Could you check a few things on this drawing? It's one solid part, dimensions in mm from its lowest x, y, z. A direction names the side the tool comes from. Round coordinates to 2 decimals unless told otherwise and drop trailing zeros. Write each loop counter-clockwise with the first axis right and the second up, starting at its lowest first coordinate (ties: lowest second). Pieces come first, ordered by that corner, then holes. Notation, with made-up numbers: (-21.75, 16) -> (24.25, 16) arc R27 cw to (24.25, 38) -> close; hole circle Ø4 at (63.25, 49). An arc over 180 degrees is marked (long way). Answer in a Markdown table with one row per item.
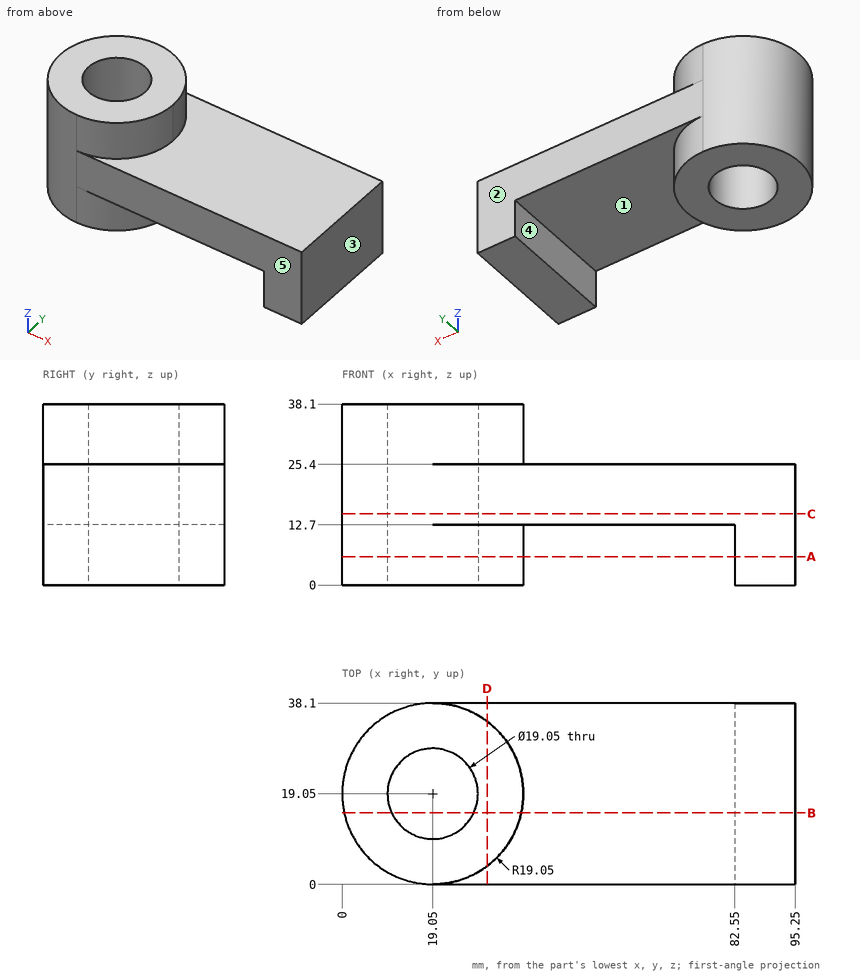
1) Please list where these lines run through material, in increasing order: line 1 (X direction, y = 19, z = 11); line 2 (Y direction, x = 19, z = 25); line 3 (X direction, y = 15, z = 3.5).
Findings:
| item | result |
|---|---|
| line 1 | x = 0 to 9.53, 28.57 to 38.1, 82.55 to 95.25 |
| line 2 | y = 0 to 9.53, 28.57 to 38.1 |
| line 3 | x = 0.44 to 10.43, 27.67 to 37.66, 82.55 to 95.25 |
2) Imagine slicing it at D-D, the plane x = 30.5. Please give me the cut outline in (y, z).
Findings:
| item | result |
|---|---|
| outline | (0, 12.7) -> (3.83, 12.7) -> (3.83, 0) -> (34.27, 0) -> (34.27, 12.7) -> (38.1, 12.7) -> (38.1, 25.4) -> (34.27, 25.4) -> (34.27, 38.1) -> (3.83, 38.1) -> (3.83, 25.4) -> (0, 25.4) -> close |
3) Imagine slicing it at C-C, the plane z = 15. Please give me the cut outline in (x, y) (3 decimals), plus the area to 3 significant figures.
Findings:
| item | result |
|---|---|
| outline | (19.05, 0) -> (95.25, 0) -> (95.25, 38.1) -> (19.05, 38.1) arc R19.05 ccw to start; hole circle Ø19.05 at (19.05, 19.05) |
| area | 3,190 mm^2 |
4) For pin 1 (4 mm diameter, centred on y = 28, z = 7, fed in from -X); pin 2 (5 mm diameter, centred on y = 5, z = 24, fed in from -X); pin 3 (3 mm diameter, centred on y = 26.5, z = 25.5, fed in from -X), each with a flat end and sliding along its axis, tell me the tip position at first contact or that it passes through.
Findings:
| item | result |
|---|---|
| pin 1 | stops at x = 1.31 |
| pin 2 | stops at x = 3.9 |
| pin 3 | stops at x = 0.95 |
5) Imagine slicing it at A-A, the plane z = 6. Please give me the cut outline in (x, y) (3 decimals).
Findings:
| item | result |
|---|---|
| outline | (19.05, 0) arc R19.05 ccw to (38.1, 19.05) arc R19.05 ccw (long way) to start; (82.55, 0) -> (95.25, 0) -> (95.25, 38.1) -> (82.55, 38.1) -> close; hole circle Ø19.05 at (19.05, 19.05) |
6) For the marked faces 4 and 5, which set-ups out of +Z, -Z, +X, -X, +Y, -Y let a thin tool reach every point of the face, with its end or its side?
Findings:
| item | result |
|---|---|
| face 4 | -Z, +Y, -Y |
| face 5 | +Z, -Z, +X, -X, -Y |
7) Thinking about a two-plate mould opening in X: for the marked faces 1, 2 and 3, which applies, +X half, -X half, draft (parallel to the pull), parting line (faces both ways), or undercut?
Findings:
| item | result |
|---|---|
| face 1 | undercut |
| face 2 | draft |
| face 3 | +X half |
8) Imagine slicing it at B-B, the plane y = 15. Please give me the cut outline in (x, z).
Findings:
| item | result |
|---|---|
| outline | (0.44, 0) -> (10.43, 0) -> (10.43, 38.1) -> (0.44, 38.1) -> close; (27.67, 0) -> (37.66, 0) -> (37.66, 12.7) -> (82.55, 12.7) -> (82.55, 0) -> (95.25, 0) -> (95.25, 25.4) -> (37.66, 25.4) -> (37.66, 38.1) -> (27.67, 38.1) -> close |
